Verification items for the finished model (mm, model axes). A direction names the side the tool comes from. Coordinates: 2 decimals unless noted, no trailing zeros. Write each loop counter-clockwise with the first axis right and the second up, starting at its lowest first coordinate (ties: lowest second). Pieces come first, ordered by that corner, then holes. Notation, with made-up numbers: (32.25, -29.5) - (78.25, -29.5) arc R12 ccw to (78.25, -7.5) - close; hole circle Ø10 at (-13.75, 21). An arc over 180 degrees is marked (long way). Use CSV: the item, a comma, the result in double quotes. Start each with the question number.
```python
from build123d import *

# Parameters (mm, degrees)
SZKIC2_R                    = 1.75
DODANIE_WYCI_GNI_CIE1_DEPTH = 5
SZKIC3_W                    = 36.8
SZKIC3_H                    = 5
DODANIE_WYCI_GNI_CIE2_DEPTH = 72.2
SFAZOWANIE1_SIZE            = 4


with BuildPart() as part:
    # Szkic2 → Dodanie-wyciągnięcie1 (new body)
    with BuildSketch(Plane.XZ.offset(-37.529198257)):
        with BuildLine():
            Line((76.54438393, 616.406662223), (39.74438393, 616.406662223))
            Line((39.74438393, 616.406662223), (39.74438393, 589.406662223))
            ThreePointArc((39.74438393, 589.406662223), (58.14438393, 571.006662223), (76.54438393, 589.406662223))
            Line((76.54438393, 589.406662223), (76.54438393, 616.406662223))
        make_face()
        with Locations(Location((50.39438393, 575.983268464, 0), (0, 0, 270))):
            Circle(SZKIC2_R, mode=Mode.SUBTRACT)
        with Locations(Location((65.89438393, 575.983268464, 0), (0, 0, 270))):
            Circle(SZKIC2_R, mode=Mode.SUBTRACT)
        with Locations(Location((73.64438393, 589.406662223, 0), (0, 0, 270))):
            Circle(SZKIC2_R, mode=Mode.SUBTRACT)
        with Locations(Location((65.89438393, 602.830055981, 0), (0, 0, 270))):
            Circle(SZKIC2_R, mode=Mode.SUBTRACT)
        with Locations(Location((50.39438393, 602.830055981, 0), (0, 0, 270))):
            Circle(SZKIC2_R, mode=Mode.SUBTRACT)
        with Locations(Location((42.64438393, 589.406662223, 0), (0, 0, 270))):
            Circle(SZKIC2_R, mode=Mode.SUBTRACT)
    extrude(amount=DODANIE_WYCI_GNI_CIE1_DEPTH)

    # Szkic3 → Dodanie-wyciągnięcie2 (add)
    with BuildSketch(Plane.XZ.offset(-32.529198257)):
        with Locations((58.14438393, 613.906662223)):
            Rectangle(SZKIC3_W, SZKIC3_H)
    extrude(amount=DODANIE_WYCI_GNI_CIE2_DEPTH)

    # Sfazowanie1
    sfazowanie1_edges = [part.edges().sort_by_distance(p)[0] for p in [
        (58.14438393, 32.529198257, 611.406662223),
    ]]
    chamfer(sfazowanie1_edges, length=SFAZOWANIE1_SIZE)


solid = part.part
```
Q1. Cross-section at A-A (x = 49.5). Record the cut outline in (y, z).
Q2. Cross-section at D-D (y = -21). Record the cut outline in (x, z).
Q3. Scan lines: line 1 along Y through (x, z) = (68, 576); line 2 along Z through (x, y) = (74, 6); line 3 along Y through (x, z) = (56, 608). Record each from-to range of solid material in increasing order. Write a range as from..to.
Q4. Gauge pin test, flat ends, axial feed: pin 1 (2 mm diameter, centred on x = 67, y = 14.5, fed in from -Z); pin 2 (2 mm diameter, centred on x = 55.5, y = 28.5, fed in from -Z); pin 3 (2 mm diameter, centred on x = 73.64, z = 589.41, fed in from -Y); pin 4 (12 mm diameter, centred on y = -22.5, z = 607.5, fed in from +X). Record the tip position at first contact, or that the pin passes through.
Q5. Release check for a two-part mould opening along Z. For faces 3 (the cylindrical face through (57.74, 35.06, 571.01)), 4 (the cylindrical face through (50.47, 35.06, 577.73)), 5 (the flat face through (39.744, 8, 612)) record: released by +Z, released by -Z, zero draft, split by the parting line, or undercut.
Q6. Cross-section at C-C (z = 595.5). Record the cut outline in (x, y), plus the area to 3 significant figures.
Q7. Cross-section at B-B (x = 70). Record the cut outline in (y, z).
Q8. Tool access check on faces 1 (the flat face through (58, 32.529, 589)), 2 (the cylindrical face through (66.42, 35.06, 601.16)). Record the directions out of +Z, -Z, +X, -X, +Y, -Y that give a thin tool (end or side, any length) a straight path to the whole face; none if there is none.
Reply:
1,outline,"(-39.67, 611.41) - (28.53, 611.41) - (32.53, 607.41) - (32.53, 604.33) - (37.53, 604.33) - (37.53, 616.41) - (-39.67, 616.41) - close; (32.53, 573.16) - (37.53, 573.16) - (37.53, 574.48) - (32.53, 574.48) - close; (32.53, 577.49) - (37.53, 577.49) - (37.53, 601.33) - (32.53, 601.33) - close"
2,outline,"(39.74, 611.41) - (76.54, 611.41) - (76.54, 616.41) - (39.74, 616.41) - close"
3,line 1,"32.53..37.53"
3,line 2,"611.41..616.41"
3,line 3,"31.94..37.53"
4,pin 1,"z = 611.41"
4,pin 2,"z = 610.44"
4,pin 3,"through"
4,pin 4,"x = 76.54"
5,face 3,"released by -Z"
5,face 4,"undercut"
5,face 5,"zero draft"
6,outline,"(39.74, 32.53) - (76.54, 32.53) - (76.54, 37.53) - (39.74, 37.53) - close"
6,area,"184 mm^2"
7,outline,"(-39.67, 611.41) - (28.53, 611.41) - (32.53, 607.41) - (32.53, 575.34) - (37.53, 575.34) - (37.53, 616.41) - (-39.67, 616.41) - close"
8,face 1,"-Z, +X, -X, -Y"
8,face 2,"+Y, -Y"
